from build123d import *

# Parameters (mm, degrees)
BASENUT_DEPTH = 16
GRVSKE_W      = 7
GRVSKE_H      = 2.75
DOMEFILLET_R  = 1


with BuildPart() as part:
    # BaseNutSke → BaseNut (new body)
    with BuildSketch(Plane(origin=(0, 0, 0), x_dir=(0, 0, -1), z_dir=(1, 0, 0))):
        Polygon((13.5, 7.794228634), (13.5, -7.794228634), (0, -15.588457268), (-13.5, -7.794228634), (-13.5, 7.794228634), (0, 15.588457268), align=None)
    extrude(amount=BASENUT_DEPTH)

    # DomeSke → Dome (revolve)
    with BuildSketch(Plane.XY):
        with BuildLine():
            Line((34, 0), (0, 0))
            Line((0, 0), (0, 12))
            Line((0, 12), (22, 12))
            ThreePointArc((22, 12), (30.485281374, 8.485281374), (34, 0))
        make_face()
    revolve(axis=Axis((0, 0, 0), (1, 0, 0)))

    # Sketch4 → DoubleChamfer (revolve, cut)
    with BuildSketch(Plane.XY, mode=Mode.PRIVATE) as doublechamfer_sk:
        Polygon((0, 13.5), (2.504809472, 17.838457268), (13.495190528, 17.838457268), (16, 13.5), (18, 13.5), (18, 28.5), (-2, 28.5), (-2, 13.5), align=None)
    revolve(doublechamfer_sk.sketch.rotate(Axis((0, 0, 0), (1, 0, 0)), 90), axis=Axis((0, 0, 0), (1, 0, 0)), mode=Mode.SUBTRACT)

    # TapDriSke → TapDrill (revolve, cut)
    with BuildSketch(Plane.XY, mode=Mode.PRIVATE) as tapdrill_sk:
        Polygon((0, 8.75), (27, 8.75), (32.257530416, 0), (0, 0), align=None)
    revolve(tapdrill_sk.sketch.rotate(Axis((0, 0, 0), (1, 0, 0)), 90), axis=Axis((0, 0, 0), (1, 0, 0)), mode=Mode.SUBTRACT)

    # GrvSke → Groove (revolve, cut)
    with BuildSketch(Plane.XY, mode=Mode.PRIVATE) as groove_sk:
        with Locations((19.5, 9.125)):
            Rectangle(GRVSKE_W, GRVSKE_H)
    revolve(groove_sk.sketch.rotate(Axis((0, 0, 0), (1, 0, 0)), 90), axis=Axis((0, 0, 0), (1, 0, 0)), mode=Mode.SUBTRACT)

    # EndChamferSketch → EndChamfer (revolve, cut)
    with BuildSketch(Plane.XY, mode=Mode.PRIVATE) as endchamfer_sk:
        Polygon((-0.0254, 10), (0.0254, 10), (0.988185365, 8.625), (-0.0254, 8.625), align=None)
    revolve(endchamfer_sk.sketch.rotate(Axis((0, 0, 0), (-1, 0, 0)), 270), axis=Axis((0, 0, 0), (-1, 0, 0)), mode=Mode.SUBTRACT)

    # DomeFillet
    domefillet_edges = [part.edges().sort_by_distance(p)[0] for p in [
        (16, -12, 0),
    ]]
    fillet(domefillet_edges, radius=DOMEFILLET_R)


solid = part.part
Read the model definition and answer for the solid it produces. Units are mm, in the model's axes. A direction names the side the tool comes from. Give positions to 0.01 mm unless a question says otherwise; leave off trailing zeros. Write each loop counter-clockwise with the first axis right and the second up, starting at its lowest first coordinate (ties: lowest second). Pieces come first, ordered by that corner, then holes. Notation, with made-up numbers: (40, 8.5) - (51, 8.5) arc R31 cw to (51, 44.5) - close; hole circle Ø2 at (34, 1.25). An arc over 180 degrees is marked (long way). Return JSON: item names as keys, results as strings.
Q1. Given P1, Ø10, axis at y = -1.5, z = 10.5, coming from the -X side; P2, Ø12, axis at x = 29, z = 2, coming from the -Y side; P3, Ø4, axis at x = 26, y = 8.5, coming from the +Z side; P4, Ø10.5, axis at y = 2, z = -1.5, coming from the -X side, each flat-ended and moving along its own axis, determine where each tip first touches the part or whether it passes through.
Reply:
{"P1": "x = 0", "P2": "y = -11.93", "P3": "z = 9.45", "P4": "x = 27.6"}
Q2. A cutting plane is placed at A-A, the plane x = 12. Determine the outline of the cut face in (y, z).
Reply:
{"outline": "(-15.59, 0) - (-7.79, -13.5) - (7.79, -13.5) - (15.59, 0) - (7.79, 13.5) - (-7.79, 13.5) - close; hole circle Ø17.5 at (0, 0)"}
Q3. For faces 1 (the face through (7.888, -11.746, 6.656)), 2 (the face through (19.54, -11.99, 0.53)), determine the directions among +Z, -Z, +X, -X, +Y, -Y from which every point of the face is accessible in a straight line to the end or side of a thin tool.
Reply:
{"face 1": "+Z, +X, -X, -Y", "face 2": "+X"}
Q4. For a pull along X with two mould halves and no side action, classify faces 3 (the face through (16, -8, 4)), 4 (the face through (23, -8, 4)), 5 (the face through (0.293, -14.008, 0.034)), 6 (the face through (8.56, 8.54, -1.9)) as released by +X, released by -X, zero draft, split by the parting line, or undercut.
Reply:
{"face 3": "undercut", "face 4": "undercut", "face 5": "released by -X", "face 6": "zero draft"}
Q5. Consider line 1 along Y through (x, z) = (10, 0); line 2 along X through (y, z) = (-11, 7.25); line 3 along Y through (x, z) = (25.1, 0). Determine where each line is inside the solid, lowest interval first. Write a range as [from, to].
Reply:
{"line 1": "[-15.59, -8.75], [8.75, 15.59]", "line 2": "[0, 16]", "line 3": "[-11.59, -8.75], [8.75, 11.59]"}
